Work out the finished part from the listing and answer in its coordinate system (mm). Face numbers are marked on the shaded views. A direction names the side the tool comes from. Give positions to 0.01 mm unless a question says otherwise; leave off trailing zeros. Loops run counter-clockwise (first coordinate to the right, second up) from the corner with the lowest first, then second, coordinate; pieces in that order, holes last. Notation, with made-up numbers: (-27.5, -39.75) - (25.5, -39.75) arc R35 cw to (25.5, -1.75) - close; hole circle Ø6 at (85, 40.25). An arc over 180 degrees is marked (long way). One line per item, written item: value.
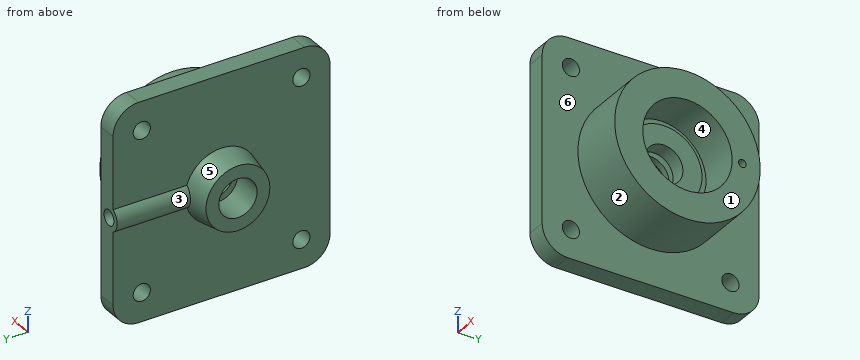
from build123d import *

# Parameters (mm, degrees)
SKETCH_2_R          = 6.75
SKETCH_2_R_2        = 20
EXTRUDE_1_DEPTH     = 15
EXTRUDE_2_REACH     = 208.216
SKETCH_3_R          = 10
SKETCH_6_R          = 3
CUT_EXTRUDE_1_DEPTH = 33
SKETCH_8_R          = 3
CUT_EXTRUDE_2_DEPTH = 58
EXTRUDE_START       = 6
EXTRUDE_3_DEPTH     = 6
EXTRUDE_4_DEPTH     = 58


with BuildPart() as part:
    # Эскиз1 → Повернуть1 (revolve)
    with BuildSketch(Plane.XY, mode=Mode.PRIVATE) as revolve_1_sk:
        Polygon((0, -15), (0, -25), (20, -28.526539614), (20, -57), (80, -57), (80, -35), (48, -35), (48, -30), (51, -30), (51, -15), (39, -15), (39, -20), (34, -20), (34, -15), (29, -15), (29, -20), (24, -20), (24, -15), align=None)
    revolve(revolve_1_sk.sketch.rotate(Axis((-987.033440026, 0, 0), (1, 0, 0)), 270), axis=Axis((-987.033440026, 0, 0), (1, 0, 0)))

    # Эскиз2 → Бобышка-Вытянуть1 (add)
    with BuildSketch(Plane.ZY.offset(-20)):
        with BuildLine():
            Line((-65, -85), (65, -85))
            ThreePointArc((65, -85), (79.142135624, -79.142135624), (85, -65))
            Line((85, -65), (85, 65))
            ThreePointArc((85, 65), (79.142135624, 79.142135624), (65, 85))
            Line((65, 85), (-65, 85))
            ThreePointArc((-65, 85), (-79.142135624, 79.142135624), (-85, 65))
            Line((-85, 65), (-85, -65))
            ThreePointArc((-85, -65), (-79.142135624, -79.142135624), (-65, -85))
        make_face()
        with Locations((-62.5, -62.5)):
            Circle(SKETCH_2_R, mode=Mode.SUBTRACT)
        with Locations((-62.5, 62.5)):
            Circle(SKETCH_2_R, mode=Mode.SUBTRACT)
        with Locations((62.5, 62.5)):
            Circle(SKETCH_2_R, mode=Mode.SUBTRACT)
        with Locations((62.5, -62.5)):
            Circle(SKETCH_2_R, mode=Mode.SUBTRACT)
        Circle(SKETCH_2_R_2, mode=Mode.SUBTRACT)
    extrude(amount=-EXTRUDE_1_DEPTH)

    # Эскиз3 → Бобышка-Вытянуть2 (add, up to next)
    with BuildSketch(Plane(origin=(0, 85, 0), x_dir=(1, 0, 0), z_dir=(0, 1, 0)), mode=Mode.PRIVATE) as extrude_2_sk1:
        with Locations((25, 0)):
            Circle(SKETCH_3_R)
    extrude_2_tool1 = extrude(extrude_2_sk1.sketch, amount=-EXTRUDE_2_REACH, mode=Mode.PRIVATE) - part.part
    add(extrude_2_tool1.solids().sort_by_distance((25, 85, 0))[0])

    # Вырез-По сечениям1: read off the stored shape, not the designer's step
    # Вырез-По сечениям1: loft between two sections, ruled curve by curve
    loft_1_from = [
        Edge.make_bspline([(25.773422165, 73, -2.898588994), (19.976244177, 73, -4.445433323), (18.429399848, 73, 1.351744665), (24.226577835, 73, 2.898588994), (30.023755823, 73, 4.445433323), (31.570600152, 73, -1.351744665), (25.773422165, 73, -2.898588994)], [0, 0, 0, 0, 0.5, 0.5, 0.5, 1, 1, 1, 1], 3, [1, 0.333333333, 0.333333333, 1, 0.333333333, 0.333333333, 1]),
    ]
    loft_1_to = [
        Edge.make_bspline([(23.045798977, 85, -5.672838651), (11.700121675, 85, -1.764436604), (15.608523722, 85, 9.581240698), (26.954201023, 85, 5.672838651), (38.299878325, 85, 1.764436604), (34.391476278, 85, -9.581240698), (23.045798977, 85, -5.672838651)], [0, 0, 0, 0, 0.5, 0.5, 0.5, 1, 1, 1, 1], 3, [1, 0.333333333, 0.333333333, 1, 0.333333333, 0.333333333, 1]),
    ]
    loft_1 = Solid(Shell([*[Face.make_surface_from_curves(loft_1_from[k], loft_1_to[k]) for k in range(1)], Face(Wire(loft_1_from)), Face(Wire(loft_1_to))]))
    add(loft_1, mode=Mode.SUBTRACT)

    # Эскиз6 → Вырез-Вытянуть1 (cut)
    with BuildSketch(Plane(origin=(0, 73, 0), x_dir=(1, 0, 0), z_dir=(0, 1, 0))):
        with Locations(Location((25, 0, 0), (0, 0, 270))):
            Circle(SKETCH_6_R)
    extrude(amount=-CUT_EXTRUDE_1_DEPTH, mode=Mode.SUBTRACT)

    # Эскиз8 → Вырез-Вытянуть2 (cut)
    with BuildSketch(Plane(origin=(80, 0, 0), x_dir=(0, 0, -1), z_dir=(1, 0, 0))):
        with Locations((0, 43)):
            Circle(SKETCH_8_R)
    extrude(amount=-CUT_EXTRUDE_2_DEPTH, mode=Mode.SUBTRACT)

    # Эскиз10 → Бобышка-Вытянуть3 (add)
    with BuildSketch(Plane(origin=(0, 40, 0), x_dir=(1, 0, 0), z_dir=(0, 1, 0)).offset(EXTRUDE_START)):
        with BuildLine():
            Line((25, 3), (25, 4.5))
            ThreePointArc((25, 4.5), (20.5, 0), (25, -4.5))
            Line((25, -4.5), (25, -3))
            ThreePointArc((25, -3), (22, 0), (25, 3))
        make_face()
    extrude(amount=-EXTRUDE_3_DEPTH)

    # Эскиз11 → Бобышка-Вытянуть4 (add)
    with BuildSketch(Plane(origin=(80, 0, 0), x_dir=(0, 0, -1), z_dir=(1, 0, 0))):
        with BuildLine():
            Line((3, 43), (4.5, 43))
            ThreePointArc((4.5, 43), (0, 38.5), (-4.5, 43))
            Line((-4.5, 43), (-3, 43))
            ThreePointArc((-3, 43), (0, 40), (3, 43))
        make_face()
    extrude(amount=-EXTRUDE_4_DEPTH)


solid = part.part
1. For the marked faces 1, 2 and 3, determine the directions among +Z, -Z, +X, -X, +Y, -Y from which every point of the face is accessible in a straight line to the end or side of a thin tool.
Output:
face 1: +Z, -Z, +X, +Y, -Y
face 2: +X
face 3: -X, +Y
2. The mould has two halves that part along Y. Classify the marked faces 4, 5 and 6: released by +Y, released by -Y, zero draft, split by the parting line, or undercut.
Output:
face 4: undercut
face 5: split by the parting line
face 6: zero draft
3. Find the intervals of material crossed by line 1 along Y through (x, z) = (58, 0); line 2 along Y through (x, z) = (28.5, 62.5); line 3 along X through (y, z) = (-11.5, 10.5), in increasing order.
Output:
line 1: y = -57 to -35, 35 to 40, 46 to 57
line 2: y = -85 to -69.25, -55.75 to 55.75, 69.25 to 85
line 3: x = 0 to 24, 29 to 34, 39 to 51
4. Section A-A (z = 62.5) is taken. Write down the section's boundary in (x, y).
Output:
outline: (20, -85) - (35, -85) - (35, -69.25) - (20, -69.25) - close; (20, -55.75) - (35, -55.75) - (35, 55.75) - (20, 55.75) - close; (20, 69.25) - (35, 69.25) - (35, 85) - (20, 85) - close
5. Flat-ended cylindrical pins translate along their axes: pin 1 Ø15.5 at (y, z) = (-62.5, 62.5) entering from +X; pin 2 Ø5.5 at (y, z) = (43, 0) entering from +X; pin 3 Ø12 at (y, z) = (32, -54) entering from +X; pin 4 Ø17.5 at (y, z) = (-62.5, -62.5) entering from -X. Find the tip coordinate at first contact, or state that the pin passes through.
Output:
pin 1: stops at x = 35
pin 2: stops at x = 23.8
pin 3: stops at x = 80
pin 4: stops at x = 20
6. Section D-D (y = -51.5) is taken. Write down the section's boundary in (x, z), and give its area (3 significant figures).
Output:
outline: (20, -85) - (35, -85) - (35, -24.43) - (80, -24.43) - (80, 24.43) - (35, 24.43) - (35, 85) - (20, 85) - close
area: 4,750 mm²
7. Section B-B (y = 62.5) is taken. Write down the section's boundary in (x, z), and give its area (3 significant figures).
Output:
outline: (20, -85) - (35, -85) - (35, -69.25) - (20, -69.25) - close; (20, -55.75) - (35, -55.75) - (35, 55.75) - (20, 55.75) - (20, 8.66) arc R10 ccw to (20, -8.66) - close; (20, 69.25) - (35, 69.25) - (35, 85) - (20, 85) - close; hole circle Ø6 at (25, 0)
area: 2,180 mm²
8. Section C-C (x = 57) is taken. Write down the section's boundary in (y, z), and give its area (3 significant figures).
Output:
outline: circle Ø114 at (0, 0); hole circle Ø70 at (0, 0); hole circle Ø6 at (43, 0)
area: 6,330 mm²
